Can you work these out from the model? Positions are in its coordinate system, mm. A direction names the side the tool comes from. Round coordinates to 2 decimals unless told otherwise and drop trailing zeros. Write each loop counter-clockwise with the first axis right and the second up, starting at its lowest first coordinate (ties: lowest second). Pieces come first, ordered by that corner, then holes. Notation, with made-up numbers: M 41.25,83.5 L 82.25,83.5 A17 ccw 82.25,87.5 Z; hole C 40.5,52 d1. An arc over 180 degrees is marked long. Answer in a Markdown table with one row per item. Add a question column.
(1) Suppose I cut it at B-B, the plane y = -1.25. Write out the boundary of the cut face in (x, z), then the cut area to 3 significant figures.
(2) For faces 1 (the face through (-0.176, -14.191, 0.286)), 2 (the face through (2.5, -4, 2)), 3 (the face through (-2.597, -13.438, 1.511)), which set-ups out of +Z, -Z, +X, -X, +Y, -Y let a thin tool reach every point of the face, with its end or its side?
(3) Suppose I cut it at C-C, the plane z = -1.5. Write out the boundary of the cut face in (x, y).
(4) If I drill on probe 1 along Y at (x, z) = (0.25, 4.75); probe 2 along Y at (x, z) = (0, 1.7); probe 3 along Z at (x, y) = (0, -13.5) (3 decimals), over which ranges is the centre line in solid material (lowest first)?
(5) If we mould it in two halves opening along Y, with no side actions, what happens to faces 4 (the face through (-3, -9.25, 2)), 5 (the face through (-0.34, -1.55, 1.6)), 6 (the face through (-3.055, -8.616, 3.968)), 7 (the face through (0, -9.25, 2))? For each: released by +Y, released by -Y, zero draft, split by the parting line, or undercut.
(6) I'm going to push flat-ended pins straight in: pin 1 (3 mm diameter, centred on y = -4, z = 2, fed in from +X); pin 2 (4 mm diameter, centred on x = -2.5, y = -3, fed in from -Z); pin 3 (4 mm diameter, centred on y = -10, z = 2, fed in from +X); pin 4 (2.5 mm diameter, centred on x = 0, y = 0, fed in from +Z). Where does each tip first touch, or does it pass through?
from build123d import *

# Parameters (mm, degrees)
SKETCH1_R           = 1.5875
BOSS_EXTRUDE1_DEPTH = 3.25


with BuildPart() as part:
    # Sketch1 → Boss-Extrude1 (new body)
    with BuildSketch(Plane.XY):
        with BuildLine():
            Line((2.5, 0), (2.5, -8))
            Line((2.5, -8), (-2.5, -8))
            Line((-2.5, -8), (-2.5, 0))
            ThreePointArc((-2.5, 0), (0, 2.5), (2.5, 0))
        make_face()
        Circle(SKETCH1_R, mode=Mode.SUBTRACT)
    extrude(amount=BOSS_EXTRUDE1_DEPTH)

    # Sketch4 one side → Revolve1 (revolve)
    with BuildSketch(Plane.XY.offset(1.625)):
        Polygon((2.6, -8), (0, -8), (0, -9.25), (1.35, -9.25), (1.35, -18.994831853), (4.6, -18.994831853), (4.6, -17.744831853), (2.6, -17.744831853), (2.6, -9.25), (3.85, -9.25), (3.85, -8), align=None)
    revolve(axis=Axis((0, -19.5, 1.625), (0, 1, 0)))


solid = part.part
Calculated:
| question | item | result |
|---|---|---|
| 1 | outline | M -2.5,0 L -0.98,0 L -0.98,3.25 L -2.5,3.25 Z; M 0.98,0 L 2.5,0 L 2.5,3.25 L 0.98,3.25 Z |
| 1 | area | 9.89 mm² |
| 2 | face 1 | -Y |
| 2 | face 2 | +Z, -Z, +X, +Y |
| 2 | face 3 | none |
| 3 | outline | M -3.38,-18.99 L 3.38,-18.99 L 3.38,-17.74 L -3.38,-17.74 Z; M -2.25,-9.25 L 2.25,-9.25 L 2.25,-8 L -2.25,-8 Z |
| 4 | probe 1 | -18.99 to -17.74, -9.25 to -8 |
| 4 | probe 2 | -9.25 to -1.59, 1.59 to 2.5 |
| 4 | probe 3 | -0.975 to 0.275, 2.975 to 4.225 |
| 5 | face 4 | undercut |
| 5 | face 5 | undercut |
| 5 | face 6 | zero draft |
| 5 | face 7 | released by -Y |
| 6 | pin 1 | x = 2.5 |
| 6 | pin 2 | z = 0 |
| 6 | pin 3 | x = 3.85 |
| 6 | pin 4 | through |
